```python
from build123d import *

# Parameters (mm, degrees)
SKETCH1_R           = 4.8
BOSS_EXTRUDE1_DEPTH = 30
SKETCH2_R           = 6.5
BOSS_EXTRUDE2_DEPTH = 4
SKETCH3_R           = 3.5
CUT_EXTRUDE1_DEPTH  = 15
CUT_EXTRUDE1_DRAFT  = -6


with BuildPart() as part:
    # Sketch1 → Boss-Extrude1 (new body)
    with BuildSketch(Plane.XY):
        Circle(SKETCH1_R)
    extrude(amount=BOSS_EXTRUDE1_DEPTH)

    # Sketch2 → Boss-Extrude2 (add)
    with BuildSketch(Plane.XY.offset(30)):
        Circle(SKETCH2_R)
    extrude(amount=BOSS_EXTRUDE2_DEPTH)


with BuildPart() as cut_extrude1_tool:
    # Sketch3 → Cut-Extrude1 (with draft: the straight prism first)
    with BuildSketch(Plane(origin=(0, 0, 0), x_dir=(-1, 0, 0), z_dir=(0, 0, -1))):
        Circle(SKETCH3_R)
    extrude(amount=-CUT_EXTRUDE1_DEPTH)
    # Cut-Extrude1: the draft: its side faces are tilted about the plane it starts from
    cut_extrude1_sides = [cut_extrude1_tool.faces().sort_by_distance(p)[0] for p in [
        (3.5, 0, 7.5),
    ]]
    draft(cut_extrude1_sides, Plane(origin=(0, 0, 0), x_dir=(-1, 0, 0), z_dir=(0, 0, -1)), CUT_EXTRUDE1_DRAFT)


with BuildPart() as part_1:
    add(part.part)

    # Cut-Extrude1: cut by cut_extrude1_tool
    add(cut_extrude1_tool.part, mode=Mode.SUBTRACT)


solid = part_1.part
```
Part model, mm, in its own coordinate system. A direction names the side the tool comes from. Give positions to 0.01 mm unless a question says otherwise; leave off trailing zeros. Order: outer loops, then holes, each group sorted by start corner. A loop starts at its lowest first (then second) coordinate and runs counter-clockwise, first axis right, second up. Notation, with made-up numbers: (88.5, 2.5) - (144.5, 2.5) arc R6 ccw to (144.5, 10.5) - close; hole circle Ø2 at (21, 26.25). An arc over 180 degrees is marked (long way). Use one line per item in the form item = value.
Item 1: Probe probe 1 along Z at (x, y) = (-1.5, -0.25); probe 2 along Z at (x, y) = (1.25, -5.75); probe 3 along Y at (x, z) = (-2.25, 6.5). List the from-to ranges inside material, lowest first. Write a range as from..to.
Solution:
probe_1 = 15..34
probe_2 = 30..34
probe_3 = -4.24..-1.69, 1.69..4.24
Item 2: Two-plate mould, pull along X, no slides. Class faces 3 (the face through (-1, -5, 30)), 4 (the face through (-5.158, -3.955, 31.972)), 5 (the face through (0, 0, 15)), 6 (the face through (2.16, -1.66, 7.4)): released by +X, released by -X, zero draft, split by the parting line, or undercut.
Solution:
face_3 = zero draft
face_4 = split by the parting line
face_5 = undercut
face_6 = undercut
Item 3: Pin check, flat tips, straight feed: pin 1 Ø1 at (x, z) = (3, 30) entering from -Y; pin 2 Ø1 at (x, z) = (3.5, 17.5) entering from -Y; pin 3 Ø1.9 at (x, y) = (0, 0.5) entering from -Z. Stop position of each tip, or through.
Solution:
pin_1 = -6
pin_2 = -3.75
pin_3 = 15
Item 4: Slice it at C-C on z = 10.5. Give the cut face in (x, y).
Solution:
outline = circle Ø9.6 at (0, 0); hole circle Ø4.79 at (0, 0)
Item 5: Which spindle directions (+Z, -Z, +X, -X, +Y, -Y) get a long thin tool onto all of the face, cutting with end or side? Do faces 1 (the face through (2.58, 4.05, 14.79)), 2 (the face through (0, -4, 0)). Say none if no direction does.
Solution:
face_1 = -Z
face_2 = -Z, +X, -X, +Y, -Y
Item 6: Slice it at A-A on x = 0. Give the cut face in (y, z), and give its area (3 significant figures).
Solution:
outline = (-6.5, 30) - (-4.8, 30) - (-4.8, 0) - (-3.5, 0) - (-1.92, 15) - (1.92, 15) - (3.5, 0) - (4.8, 0) - (4.8, 30) - (6.5, 30) - (6.5, 34) - (-6.5, 34) - close
area = 259 mm2
Item 7: Slice it at D-D on z = 26. Give the cut face in (x, y).
Solution:
outline = circle Ø9.6 at (0, 0)
